```python
from build123d import *

# Parameters (mm, degrees)
SKETCH3_R               = 7
BOSS_EXTRUDE1_DEPTH     = 19
SKETCH4_R               = 4
CUT_EXTRUDE1_DEPTH      = 19
CUT_EXTRUDE2_DEPTH      = 26.416530054
CUT_EXTRUDE2_DEPTH_BACK = 26.416530054
SKETCH5_W               = 12
SKETCH5_H               = 16.5


with BuildPart() as part:
    # Sketch2 → Revolve2 (revolve)
    with BuildSketch(Plane.XY, mode=Mode.PRIVATE) as revolve2_sk:
        Polygon((0, 0), (9, 0), (7, -22), (0, -22), align=None)
    revolve(revolve2_sk.sketch.rotate(Axis((0, 0, 0), (0, -1, 0)), 180), axis=Axis((0, 0, 0), (0, -1, 0)))

    # Sketch3 → Boss-Extrude1 (add)
    with BuildSketch(Plane(origin=(0, 0, 0), x_dir=(1, 0, 0), z_dir=(0, 1, 0))):
        with Locations(Location((0, 0, 0), (0, 0, 180))):
            Circle(SKETCH3_R)
    extrude(amount=BOSS_EXTRUDE1_DEPTH)

    # Sketch4 → Cut-Extrude1 (cut)
    with BuildSketch(Plane(origin=(0, 19, 0), x_dir=(1, 0, 0), z_dir=(0, 1, 0))):
        with Locations(Location((0, 0, 0), (0, 0, 180))):
            Circle(SKETCH4_R)
    extrude(amount=-CUT_EXTRUDE1_DEPTH, mode=Mode.SUBTRACT)

    # Sketch5 → Cut-Extrude2 (cut, two sides: drawn at the far end of the back side and taken through both)
    with BuildSketch(Plane.XY.offset(-CUT_EXTRUDE2_DEPTH_BACK)):
        with Locations((0, -11)):
            Rectangle(SKETCH5_W, SKETCH5_H)
    extrude(amount=CUT_EXTRUDE2_DEPTH + CUT_EXTRUDE2_DEPTH_BACK, mode=Mode.SUBTRACT)


solid = part.part
```
Design review of the part built by this model. Coordinates are the model's own, in mm. A direction names the side the tool comes from. Coordinates: 2 decimals unless noted, no trailing zeros. Loops run counter-clockwise (first coordinate to the right, second up) from the corner with the lowest first, then second, coordinate; pieces in that order, holes last. Notation, with made-up numbers: (69, -12) - (128, -12) arc R16 cw to (128, 18) - close; hole circle Ø5 at (-35.75, 88.5). An arc over 180 degrees is marked (long way). Use CSV: the item, a comma, the result in double quotes. Start each with the question number.
1) Consider section D-D on y = -4.5. Write out the cut boundary in (x, z), then the cut area to 3 significant figures.
2) Consider section C-C on y = 4. Write out the cut boundary in (x, z).
3) Tool access review of faces 1 (the flat face through (0, 0, 7.3)), 2 (the flat face through (-6, -11, 0)), 3 (the conical face through (6.3, -11.2, 4.9)): name each direction out of +Z, -Z, +X, -X, +Y, -Y from which nothing blocks a thin tool from reaching the whole face with its end or side.
4) For pin 1 Ø4 at (x, z) = (-1.5, 0) entering from +Y; pin 2 Ø3 at (y, z) = (-15, 1.5) entering from +X; pin 3 Ø2 at (x, y) = (-6.5, 12.5) entering from +Z, all flat-tipped, find the tip position at first contact; note any pin that passes through.
5) Consider section B-B on x = 0. Write out the cut boundary in (y, z), then the cut area to 3 significant figures.
6) Wall thickness on L1, parallel to Y at x = 5.25, z = -2.25; L2, parallel to Z at x = 0, y = 7.25; L3, parallel to Z at x = 1.5, y = 10: over which ranges is each line inside the solid? List them lowest first. Write a range as from..to.
7) Consider section A-A on z = 0. Write out the cut boundary in (x, y).
8) The part is to be moulded in two halves that separate along X. For faces 4 (the flat face through (0, -22, 0)), 5 (the cylindrical face through (0.867, 9.633, -3.905)), 6 (the cylindrical face through (-6.466, 9.367, -2.681)), say which applies: +X half, -X half, draft (parallel to the pull), parting line (faces both ways), or undercut.
Geometry says:
1,outline,"(-6, -6.15) - (-6, 6.15) arc R8.59 ccw to start; (6, -6.15) arc R8.59 ccw to (6, 6.15) - close"
1,area,"44.0 mm^2"
2,outline,"circle Ø14 at (0, 0); hole circle Ø8 at (0, 0)"
3,face 1,"+Y"
3,face 2,"+Z, -Z"
3,face 3,"-Y"
4,pin 1,"y = 0"
4,pin 2,"x = 7.72"
4,pin 3,"z = 4.33"
5,outline,"(-22, -7) - (-19.25, -7.25) - (-19.25, 7.25) - (-22, 7) - close; (-2.75, -8.75) - (0, -9) - (0, -7) - (19, -7) - (19, -4) - (0, -4) - (0, 4) - (19, 4) - (19, 7) - (0, 7) - (0, 9) - (-2.75, 8.75) - close"
5,area,"202 mm^2"
6,L1,"-22..-19.25, -2.75..19"
6,L2,"-7..-4, 4..7"
6,L3,"-6.84..-3.71, 3.71..6.84"
7,outline,"(-9, 0) - (-7, -22) - (7, -22) - (9, 0) - (7, 0) - (7, 19) - (4, 19) - (4, 0) - (-4, 0) - (-4, 19) - (-7, 19) - (-7, 0) - close; hole (-6, -19.25) - (6, -19.25) - (6, -2.75) - (-6, -2.75) - close"
8,face 4,"draft"
8,face 5,"undercut"
8,face 6,"parting line"
